from build123d import *

# Parameters (mm, degrees)
SKIZZE1_W                       = 135
SKIZZE1_H                       = 85
AUFSATZ_LINEAR_AUSTRAGEN1_DEPTH = 30
SCHALE1_T                       = -2
SKIZZE2_R                       = 6
SCHNITT_LINEAR_AUSTRAGEN1_DEPTH = 30
SCHNITT_LINEAR_AUSTRAGEN2_DEPTH = 10
VERRUNDUNG1_R                   = 3
AUFSATZ_LINEAR_AUSTRAGEN2_DEPTH = 6
VERRUNDUNG2_R                   = 3
SKIZZE5_W                       = 15
SKIZZE5_H                       = 10
AUFSATZ_LINEAR_AUSTRAGEN3_DEPTH = 6
VERRUNDUNG3_R                   = 3
SKIZZE6_R                       = 8.5
SCHNITT_LINEAR_AUSTRAGEN3_DEPTH = 5
SKIZZE7_W                       = 20
SKIZZE7_H                       = 20
AUFSATZ_LINEAR_AUSTRAGEN4_DEPTH = 6
VERRUNDUNG4_R                   = 3
M3_GEWINDEBOHRUNG1_D            = 2.5
M3_GEWINDEBOHRUNG1_DEPTH        = 8.5
M3_GEWINDEBOHRUNG1_TIP          = 0.751075774
M2_5_GEWINDEBOHRUNG1_D          = 2.05
M2_5_GEWINDEBOHRUNG1_DEPTH      = 7.25
M2_5_GEWINDEBOHRUNG1_TIP        = 0.615882135
SKIZZE12_W                      = 85
SKIZZE12_H                      = 6
SCHNITT_LINEAR_AUSTRAGEN4_DEPTH = 1
SKIZZE13_R                      = 3.2
SCHNITT_LINEAR_AUSTRAGEN5_DEPTH = 10
AUFSATZ_LINEAR_START            = -30
AUFSATZ_LINEAR_AUSTRAGEN5_DEPTH = 30
M3_GEWINDEBOHRUNG2_D            = 2.5
M3_GEWINDEBOHRUNG2_DEPTH        = 8.5
M3_GEWINDEBOHRUNG2_TIP          = 0.751075774
VERRUNDUNG5_R                   = 3


with BuildPart() as part:
    # Skizze1 → Aufsatz-Linear austragen1 (new body)
    with BuildSketch(Plane(origin=(0, 0, 0), x_dir=(1, 0, 0), z_dir=(0, 1, 0))):
        with Locations((67.5, 42.5)):
            Rectangle(SKIZZE1_W, SKIZZE1_H)
    extrude(amount=AUFSATZ_LINEAR_AUSTRAGEN1_DEPTH)

    # Schale1
    schale1_openings = [part.faces().sort_by_distance(p)[0] for p in [
        (67.5, 30, -42.5),
    ]]
    offset(amount=SCHALE1_T, openings=schale1_openings, kind=Kind.INTERSECTION)

    # Skizze2 → Schnitt-Linear austragen1 (cut)
    with BuildSketch(Plane.XY):
        with Locations((20.6, 15.94)):
            Circle(SKIZZE2_R)
        with Locations((34.9, 15.94)):
            Circle(SKIZZE2_R)
        with Locations((49.2, 15.94)):
            Circle(SKIZZE2_R)
        with Locations((63.5, 15.94)):
            Circle(SKIZZE2_R)
        with Locations((77.8, 15.94)):
            Circle(SKIZZE2_R)
    extrude(amount=-SCHNITT_LINEAR_AUSTRAGEN1_DEPTH, mode=Mode.SUBTRACT)

    # Skizze3 → Schnitt-Linear austragen2 (cut)
    with BuildSketch(Plane.XY):
        with BuildLine():
            ThreePointArc((109.082181292, 21.48963825), (111.018633773, 20.780819017), (112.040082938, 18.989474685))
            Line((112.040082938, 18.989474685), (115.04016588, 18.989308791))
            ThreePointArc((115.04016588, 18.989308791), (118.039999986, 15.989142906), (115.039834101, 12.9893088))
            Line((115.039834101, 12.9893088), (112.03975116, 12.989474694))
            ThreePointArc((112.03975116, 12.989474694), (111.018103892, 11.198243337), (109.081573032, 10.489638266))
            Line((109.081573032, 10.489638266), (102.54015207, 10.49))
            Line((102.54015207, 10.49), (95.998122837, 10.49))
            ThreePointArc((95.998122837, 10.49), (94.061631164, 11.198712153), (93.040082946, 12.99))
            Line((93.040082946, 12.99), (90.04, 12.99))
            ThreePointArc((90.04, 12.99), (87.04, 15.99), (90.04, 18.99))
            Line((90.04, 18.99), (93.040082946, 18.99))
            ThreePointArc((93.040082946, 18.99), (94.061631164, 20.781287847), (95.998122837, 21.49))
            Line((95.998122837, 21.49), (102.54015207, 21.49))
            Line((102.54015207, 21.49), (109.082181292, 21.48963825))
        make_face()
    extrude(amount=-SCHNITT_LINEAR_AUSTRAGEN2_DEPTH, mode=Mode.SUBTRACT)

    # Verrundung1
    verrundung1_edges = [part.edges().sort_by_distance(p)[0] for p in [
        (2, 16, -83),
        (2, 16, -2),
        (133, 16, -2),
        (133, 16, -83),
        (0, 15, -85),
        (135, 15, -85),
        (135, 15, 0),
        (0, 15, 0),
    ]]
    fillet(verrundung1_edges, radius=VERRUNDUNG1_R)

    # Skizze4 → Aufsatz-Linear austragen2 (add)
    with BuildSketch(Plane(origin=(0, 2, 0), x_dir=(1, 0, 0), z_dir=(0, 1, 0))):
        with BuildLine():
            Line((13, 12), (2, 12))
            Line((2, 12), (2, 5))
            ThreePointArc((2, 5), (2.878679656, 2.878679656), (5, 2))
            Line((5, 2), (16, 2))
            Line((16, 2), (16, 9))
            ThreePointArc((16, 9), (15.121320344, 11.121320344), (13, 12))
        make_face()
        with BuildLine():
            Line((119, 9), (119, 2))
            Line((119, 2), (130, 2))
            ThreePointArc((130, 2), (132.121320344, 2.878679656), (133, 5))
            Line((133, 5), (133, 12))
            Line((133, 12), (122, 12))
            ThreePointArc((122, 12), (119.878679656, 11.121320344), (119, 9))
        make_face()
    extrude(amount=AUFSATZ_LINEAR_AUSTRAGEN2_DEPTH)

    # Verrundung2
    verrundung2_edges = [part.edges().sort_by_distance(p)[0] for p in [
        (2, 5, -12),
        (16, 5, -2),
        (133, 5, -12),
        (119, 5, -2),
    ]]
    fillet(verrundung2_edges, radius=VERRUNDUNG2_R)

    # Skizze5 → Aufsatz-Linear austragen3 (add)
    with BuildSketch(Plane(origin=(0, 2, 0), x_dir=(1, 0, 0), z_dir=(0, 1, 0))):
        with Locations((9.5, 45.4)):
            Rectangle(SKIZZE5_W, SKIZZE5_H)
        with Locations((125.5, 45.4)):
            Rectangle(SKIZZE5_W, SKIZZE5_H)
    extrude(amount=AUFSATZ_LINEAR_AUSTRAGEN3_DEPTH)

    # Verrundung3
    verrundung3_edges = [part.edges().sort_by_distance(p)[0] for p in [
        (2, 5, -50.4),
        (2, 5, -40.4),
        (17, 5, -40.4),
        (17, 5, -50.4),
        (133, 5, -50.4),
        (118, 5, -50.4),
        (118, 5, -40.4),
        (133, 5, -40.4),
    ]]
    fillet(verrundung3_edges, radius=VERRUNDUNG3_R)

    # Skizze6 → Schnitt-Linear austragen3 (cut)
    with BuildSketch(Plane(origin=(0, 0, -85), x_dir=(-1, 0, 0), z_dir=(0, 0, -1))):
        with Locations((-92.5, 18)):
            Circle(SKIZZE6_R)
        with Locations(Location((-42.5, 18, 0), (0, 0, 180))):
            Circle(SKIZZE6_R)
    extrude(amount=-SCHNITT_LINEAR_AUSTRAGEN3_DEPTH, mode=Mode.SUBTRACT)

    # Skizze7 → Aufsatz-Linear austragen4 (add)
    with BuildSketch(Plane(origin=(0, 2, 0), x_dir=(1, 0, 0), z_dir=(0, 1, 0))):
        with Locations((42.5, 73)):
            Rectangle(SKIZZE7_W, SKIZZE7_H)
        with Locations((92.5, 73)):
            Rectangle(SKIZZE7_W, SKIZZE7_H)
    extrude(amount=AUFSATZ_LINEAR_AUSTRAGEN4_DEPTH)

    # Verrundung4
    verrundung4_edges = [part.edges().sort_by_distance(p)[0] for p in [
        (32.5, 5, -63),
        (52.5, 5, -63),
        (52.5, 5, -83),
        (32.5, 5, -83),
        (82.5, 5, -63),
        (102.5, 5, -63),
        (102.5, 5, -83),
        (82.5, 5, -83),
    ]]
    fillet(verrundung4_edges, radius=VERRUNDUNG4_R)

    # M3 Gewindebohrung1
    with Locations(Plane(origin=(0, 8, 0), x_dir=(1, 0, 0), z_dir=(0, 1, 0))):
        with Locations((125.5, 7.4), (9.5, 45.4), (125.5, 45.4), (9.5, 7.4)):
            Hole(M3_GEWINDEBOHRUNG1_D / 2, depth=M3_GEWINDEBOHRUNG1_DEPTH)
            with Locations((0, 0, -(M3_GEWINDEBOHRUNG1_DEPTH + M3_GEWINDEBOHRUNG1_TIP / 2))):  # 118° drill point
                Cone(0, M3_GEWINDEBOHRUNG1_D / 2, M3_GEWINDEBOHRUNG1_TIP, mode=Mode.SUBTRACT)

    # M2.5 Gewindebohrung1
    with Locations(Plane(origin=(0, 8, 0), x_dir=(1, 0, 0), z_dir=(0, 1, 0))):
        with Locations((42.5, 73), (92.5, 73)):
            Hole(M2_5_GEWINDEBOHRUNG1_D / 2, depth=M2_5_GEWINDEBOHRUNG1_DEPTH)
            with Locations((0, 0, -(M2_5_GEWINDEBOHRUNG1_DEPTH + M2_5_GEWINDEBOHRUNG1_TIP / 2))):  # 118° drill point
                Cone(0, M2_5_GEWINDEBOHRUNG1_D / 2, M2_5_GEWINDEBOHRUNG1_TIP, mode=Mode.SUBTRACT)

    # Skizze12 → Schnitt-Linear austragen4 (cut)
    with BuildSketch(Plane(origin=(0, 8, 0), x_dir=(1, 0, 0), z_dir=(0, 1, 0))):
        with Locations((66.348936769, 80)):
            Rectangle(SKIZZE12_W, SKIZZE12_H)
    extrude(amount=-SCHNITT_LINEAR_AUSTRAGEN4_DEPTH, mode=Mode.SUBTRACT)

    # Skizze13 → Schnitt-Linear austragen5 (cut)
    with BuildSketch(Plane(origin=(0, 2, 0), x_dir=(1, 0, 0), z_dir=(0, 1, 0))):
        with Locations(Location((97.5, 25, 0), (0, 0, 270))):
            Circle(SKIZZE13_R)
        with Locations(Location((37.5, 25, 0), (0, 0, 90))):
            Circle(SKIZZE13_R)
    extrude(amount=-SCHNITT_LINEAR_AUSTRAGEN5_DEPTH, mode=Mode.SUBTRACT)

    # Skizze14 → Aufsatz-Linear austragen5 (add)
    with BuildSketch(Plane.XZ.offset(AUFSATZ_LINEAR_START)):
        with BuildLine():
            Line((0, -85), (-4, -85))
            Line((-4, -85), (-4, 0))
            Line((-4, 0), (0, 0))
            Line((0, 0), (3, 0))
            ThreePointArc((3, 0), (0.878679656, -0.878679656), (0, -3))
            Line((0, -3), (0, -82))
            ThreePointArc((0, -82), (0.878679656, -84.121320344), (3, -85))
            Line((3, -85), (0, -85))
        make_face()
        with BuildLine():
            Line((135, 0), (139, 0))
            Line((139, 0), (139, -85))
            Line((139, -85), (135, -85))
            Line((135, -85), (132, -85))
            ThreePointArc((132, -85), (134.121320344, -84.121320344), (135, -82))
            Line((135, -82), (135, -3))
            ThreePointArc((135, -3), (134.121320344, -0.878679656), (132, 0))
            Line((132, 0), (135, 0))
        make_face()
    extrude(amount=AUFSATZ_LINEAR_AUSTRAGEN5_DEPTH)

    # M3 Gewindebohrung2
    with Locations(Plane(origin=(76.74477579, 30, -27.1140539), x_dir=(1, 0, 0), z_dir=(0, 1, 0))):
        with Locations((-76.74477579, -23.1140539), (58.25522421, 53.8859461), (-76.74477579, 53.8859461), (58.25522421, -23.1140539)):
            Hole(M3_GEWINDEBOHRUNG2_D / 2, depth=M3_GEWINDEBOHRUNG2_DEPTH)
            with Locations((0, 0, -(M3_GEWINDEBOHRUNG2_DEPTH + M3_GEWINDEBOHRUNG2_TIP / 2))):  # 118° drill point
                Cone(0, M3_GEWINDEBOHRUNG2_D / 2, M3_GEWINDEBOHRUNG2_TIP, mode=Mode.SUBTRACT)

    # Verrundung5
    verrundung5_edges = [part.edges().sort_by_distance(p)[0] for p in [
        (-4, 15, -85),
        (-4, 15, 0),
        (139, 15, 0),
        (139, 15, -85),
    ]]
    fillet(verrundung5_edges, radius=VERRUNDUNG5_R)


solid = part.part
Work out the finished part from the listing and answer in its coordinate system (mm). A direction names the side the tool comes from. Give positions to 0.01 mm unless a question says otherwise; leave off trailing zeros. Loops run counter-clockwise (first coordinate to the right, second up) from the corner with the lowest first, then second, coordinate; pieces in that order, holes last. Notation, with made-up numbers: (45, 36.5) - (61, 36.5) arc R17 cw to (61, 67.5) - close; hole circle Ø3 at (-14, -23.75). An arc over 180 degrees is marked (long way). Answer in a Markdown table with one row per item. Add a question column.
Q1. The part is cut by section D-D (z = -32). Determine the outline of the cut face in (x, y), and give its area (3 significant figures).
Q2. Consider line 1 along X through (y, z) = (2.25, -45.4); line 2 along X through (y, z) = (6, -7.4); line 3 along Z through (x, y) = (107, 7). Determine where each line is inside the solid, lowest interval first.
Q3. Determine the mould class of faces 3 (the flat face through (67.8, 30, -83.2)), 4 (the cylindrical face through (57.506, 16.204, -0.986)), 5 (the cylindrical face through (31.6, 4.54, -82.14)) for opening direction Y: released by +Y, released by -Y, zero draft, split by the parting line, or undercut.
Q4. Each of these flat-tipped pins is pushed along its axis until it touches: P1, Ø3, axis at x = 9.5, z = -45.4, coming from the +Y side; P2, Ø10, axis at x = 83, z = -36.5, coming from the +Y side. Where does it stop, or does it pass through?
Q5. The part is cut by section C-C (y = 5.5). State how many separate pieces and enclosed holes the cut face has, and give its area (3 significant figures).
Q6. A tool of negligible diameter and unlimited length cuts with its end or side. For faces 1 (the cylindrical face through (138.1, 14.79, -84.14)), 2 (the cylindrical face through (16.14, 5.04, -49.5)), from which of +Z, -Z, +X, -X, +Y, -Y can it reach the whole face along a straight path? Write none if from no direction.
Q7. The part is cut by section A-A (x = 20.6). Determine the outline of the cut face in (y, z).
Q8. The part is cut by section B-B (x = 37.5). Determine the outline of the cut face in (y, z), and give its area (3 significant figures).
Solution:
| question | item | result |
|---|---|---|
| 1 | outline | (-4, 0) - (139, 0) - (139, 30) - (133, 30) - (133, 2) - (2, 2) - (2, 30) - (-4, 30) - close |
| 1 | area | 622 mm² |
| 2 | line 1 | x = -4 to 8.25, 10.75 to 17, 118 to 124.25, 126.75 to 139 |
| 2 | line 2 | x = -4 to 8.25, 10.75 to 16, 119 to 124.25, 126.75 to 139 |
| 2 | line 3 | z = -85 to -83, -2 to 0 |
| 3 | face 3 | released by +Y |
| 3 | face 4 | undercut |
| 3 | face 5 | zero draft |
| 4 | P1 | stops at y = 8 |
| 4 | P2 | stops at y = 2 |
| 5 | separate pieces | 1 |
| 5 | enclosed holes | 7 |
| 5 | area | 2,900 mm² |
| 6 | face 1 | -Z, +X, +Y, -Y |
| 6 | face 2 | +Y |
| 7 | outline | (0, -85) - (30, -85) - (30, -83) - (2, -83) - (2, -2) - (9.94, -2) - (9.94, 0) - (0, 0) - close; (21.94, -2) - (30, -2) - (30, 0) - (21.94, 0) - close |
| 8 | outline | (0, -85) - (11.13, -85) - (11.13, -83) - (7, -83) - (7, -77) - (8, -77) - (8, -63) - (2, -63) - (2, -28.2) - (0, -28.2) - close; (0, -21.8) - (2, -21.8) - (2, -2) - (10.53, -2) - (10.53, 0) - (0, 0) - close; (21.35, -2) - (30, -2) - (30, 0) - (21.35, 0) - close; (24.87, -85) - (30, -85) - (30, -83) - (24.87, -83) - close |
| 8 | area | 334 mm² |
